```python
from build123d import *

# Parameters (mm, degrees)
F0_W           = 95
F0_H           = 65
F1_DEPTH       = 10
F3_DEPTH       = 50
F4_R           = 8
F5_R           = 4.99999
F7_D           = 7
F7_CSINK_D     = 10
F7_CSINK_ANGLE = 90
F8_T1_DEPTH    = 30
F8_T4_ANGLE    = 90
F8_T6_ANGLE    = 90
F8_T8_ANGLE    = 90
F8_T10_ANGLE   = 90


# Not quite as in the source:
# - a fillet or chamfer that OpenCascade refuses, or shapes differently, is made with other operations: its cross-section is extruded or revolved along the edge and cut away or added
# - a fillet or chamfer is up to 0.001 mm smaller than in the source, because OpenCascade refuses the exact size


with BuildPart() as f1:
    # F0 (on Top) → F1 (new body)
    with BuildSketch(Plane.XY):
        with Locations((47.5, 32.5)):
            Rectangle(F0_W, F0_H)
    extrude(amount=F1_DEPTH)

    # F2 (on face) → F3 (join)
    with BuildSketch(Plane.XY.offset(10)):
        Polygon((36, 65), (26, 65), (26, 0), (68, 0), (68, 65), (58, 65), (58, 10), (36, 10), align=None)
    extrude(amount=F3_DEPTH)

    # F4
    f4_edges = [f1.edges().sort_by_distance(p)[0] for p in [
        (68, 32.5, 10),
        (26, 32.5, 10),
    ]]
    fillet(f4_edges, radius=F4_R)

    # F5 (radius 5 in the source; OpenCascade refuses exactly that, so slightly less here)
    f5_edges = [f1.edges().sort_by_distance(p)[0] for p in [
        (85.5, 65, 10),
        (76, 32.5, 10),
        (95, 32.5, 10),
        (85.5, 0, 10),
        (9, 65, 10),
        (18, 32.5, 10),
        (0, 32.5, 10),
        (9, 0, 10),
        (31, 65, 60),
        (26, 32.5, 60),
        (47, 0, 60),
        (68, 32.5, 60),
        (63, 65, 60),
        (58, 37.5, 60),
        (47, 10, 60),
        (36, 37.5, 60),
    ]]
    fillet(f5_edges, radius=F5_R)

    # F7 (through all)
    with Locations(Plane.XY.offset(10)):
        with Locations((13, 50), (13, 15), (82, 50), (82, 15)):
            CounterSinkHole(F7_D / 2, F7_CSINK_D / 2, counter_sink_angle=F7_CSINK_ANGLE)

    # F8: fillet of radius 8 on 4 edges, made by hand

    # F8_s2 → F8_t1 (cut)
    with BuildSketch(Plane.XY.offset(-20)):
        with BuildLine():
            ThreePointArc((8, 65), (2.3431457505, 62.6568542495), (0, 57))
            Line((0, 57), (0, 65))
            Line((0, 65), (8, 65))
        make_face()
        with BuildLine():
            ThreePointArc((87, 65), (92.6568542495, 62.6568542495), (95, 57))
            Line((95, 57), (95, 65))
            Line((95, 65), (87, 65))
        make_face()
        with BuildLine():
            ThreePointArc((95, 8), (92.6568542495, 2.3431457505), (87, 0))
            Line((87, 0), (95, 0))
            Line((95, 0), (95, 8))
        make_face()
        with BuildLine():
            ThreePointArc((0, 8), (2.3431457505, 2.3431457505), (8, 0))
            Line((8, 0), (0, 0))
            Line((0, 0), (0, 8))
        make_face()
    extrude(amount=F8_T1_DEPTH, mode=Mode.SUBTRACT)

    # F8_s3 → F8_t4 (revolve, cut)
    with BuildSketch(Plane.XZ.offset(-8)):
        with BuildLine():
            ThreePointArc((4.99999, 10), (1.4644631651, 8.5355368349), (0, 5.00001))
            Line((0, 5.00001), (0, 10))
            Line((0, 10), (4.99999, 10))
        make_face()
    revolve(axis=Axis((8, 8, 10), (0, 0, 1)), revolution_arc=F8_T4_ANGLE, mode=Mode.SUBTRACT)

    # F8_s5 → F8_t6 (revolve, cut)
    with BuildSketch(Plane.YZ.offset(87)):
        with BuildLine():
            ThreePointArc((4.99999, 10), (1.4644631651, 8.5355368349), (0, 5.00001))
            Line((0, 5.00001), (0, 10))
            Line((0, 10), (4.99999, 10))
        make_face()
    revolve(axis=Axis((87, 8, 10), (0, 0, 1)), revolution_arc=F8_T6_ANGLE, mode=Mode.SUBTRACT)

    # F8_s7 → F8_t8 (revolve, cut)
    with BuildSketch(Plane.XZ.offset(-57)):
        with BuildLine():
            ThreePointArc((90.00001, 10), (93.5355368349, 8.5355368349), (95, 5.00001))
            Line((95, 5.00001), (95, 10))
            Line((95, 10), (90.00001, 10))
        make_face()
    revolve(axis=Axis((87, 57, 10), (0, 0, 1)), revolution_arc=F8_T8_ANGLE, mode=Mode.SUBTRACT)

    # F8_s9 → F8_t10 (revolve, cut)
    with BuildSketch(Plane.YZ.offset(8)):
        with BuildLine():
            ThreePointArc((60.00001, 10), (63.5355368349, 8.5355368349), (65, 5.00001))
            Line((65, 5.00001), (65, 10))
            Line((65, 10), (60.00001, 10))
        make_face()
    revolve(axis=Axis((8, 57, 10), (0, 0, 1)), revolution_arc=F8_T10_ANGLE, mode=Mode.SUBTRACT)


solid = f1.part
```
Here's how the part is built. I have some questions about the finished solid (model axes, mm). A direction names the side the tool comes from. Give positions to 0.01 mm unless a question says otherwise; leave off trailing zeros. Order: outer loops, then holes, each group sorted by start corner. A loop starts at its lowest first (then second) coordinate and runs counter-clockwise, first axis right, second up. Notation, with made-up numbers: (5.25, 7.5) - (22.25, 7.5) arc R31 cw to (22.25, 31.5) - close; hole circle Ø1 at (-36, 47.5). An arc over 180 degrees is marked (long way). Answer as a JSON object with one key per item and string values. Group by question number.
Item 1: If we section it at A-A on x = 82: Please give me the cut outline in (y, z), and give its area (3 significant figures).
Item 2: Please list where these lines run through material, in increasing order: probe 1 along X at (y, z) = (50, 2.5); probe 2 along Y at (x, z) = (82, 5.25); probe 3 along X at (y, z) = (23.5, 38).
Item 3: Which directions (+Z, -Z, +X, -X, +Y, -Y) give clear straight access to the entire face, cutting with the end or side of a thin tool? Please do faces 1 (the cylindrical face through (27, 63, 37)), 2 (the cylindrical face through (82, 63, 9)), 3 (the flat face through (26, 33, 36)), 4 (the flat face through (47, 10, 32)).
Item 4: If we mould it in two halves opening along Y, with no side actions, what happens to faces 5 (the flat face through (47, 65, 9)), 6 (the flat face through (47, 38, 10)), 7 (the conical face through (86, 15, 9))? For each: pulls with the +Y half, pulls with the -Y half, needs draft (parallel to the pull), parting line crosses it, or undercut.
Item 5: For P1, Ø4, axis at y = 23.5, z = 16, coming from the +X side; P2, Ø1.5, axis at y = 37, z = 40.5, coming from the -X side; P3, Ø8, axis at x = 82, y = 50, coming from the +Z side, each with a flat end and sliding along its axis, tell me the tip position at first contact or that it passes through.
Item 6: If we section it at C-C on z = 45: Please give me the cut outline in (x, y).
Result set:
{
 "1": {"outline": "(0, 0) - (11.5, 0) - (11.5, 8.5) - (10, 10) - (5, 10) arc R5 ccw to (0, 5) - close; (18.5, 0) - (46.5, 0) - (46.5, 8.5) - (45, 10) - (20, 10) - (18.5, 8.5) - close; (53.5, 0) - (65, 0) - (65, 5) arc R5 ccw to (60, 10) - (55, 10) - (53.5, 8.5) - close", "area": "495 mm²"},
 "2": {"probe 1": "0 to 9.5, 16.5 to 78.5, 85.5 to 95", "probe 2": "0.01 to 11.5, 18.5 to 46.5, 53.5 to 64.99", "probe 3": "26 to 36, 58 to 68"},
 "3": {"face 1": "+Z, -X, +Y", "face 2": "+Z, +X, +Y", "face 3": "+Z, -X, +Y, -Y", "face 4": "+Z, +Y"},
 "4": {"face 5": "pulls with the +Y half", "face 6": "needs draft", "face 7": "undercut"},
 "5": {"P1": "x = 69.07", "P2": "x = 26", "P3": "z = 9"},
 "6": {"outline": "(26, 5) arc R5 ccw to (31, 0) - (63, 0) arc R5 ccw to (68, 5) - (68, 60) arc R5 ccw to (63, 65) - (58, 65) - (58, 10) - (36, 10) - (36, 65) - (31, 65) arc R5 ccw to (26, 60) - close"}
}
